```python
from build123d import *

# Parameters (mm, degrees)
SKETCH_1_W          = 24
SKETCH_1_H          = 40
SKETCH_1_R          = 2
EXTRUDE_1_DEPTH     = 5
EXTRUDE_5_DEPTH     = 67.34
SKETCH_10_W         = 10
SKETCH_10_H         = 28
EXTRUDE_6_DEPTH     = 18.5
SKETCH_12_R         = 2
CUT_EXTRUDE_4_DEPTH = 24.5
SKETCH_13_W         = 12
SKETCH_13_H         = 28
CUT_EXTRUDE_5_DEPTH = 2


with BuildPart() as part:
    # 草图1 → 凸台-拉伸1 (new body)
    with BuildSketch(Plane(origin=(0, 0, 0), x_dir=(1, 0, 0), z_dir=(0, 1, 0))):
        Rectangle(SKETCH_1_W, SKETCH_1_H)
        with Locations((7.5, -14.8)):
            Circle(SKETCH_1_R, mode=Mode.SUBTRACT)
        with Locations((-7.5, -14.8)):
            Circle(SKETCH_1_R, mode=Mode.SUBTRACT)
        with Locations((-7.5, 14.8)):
            Circle(SKETCH_1_R, mode=Mode.SUBTRACT)
        with Locations((7.5, 14.8)):
            Circle(SKETCH_1_R, mode=Mode.SUBTRACT)
    extrude(amount=EXTRUDE_1_DEPTH)

    # 草图8 → 凸台-拉伸5 (add)
    with BuildSketch(Plane(origin=(0, 5, 0), x_dir=(1, 0, 0), z_dir=(0, 1, 0))):
        Polygon((-5, 0), (-5, -20), (5, -20), (5, 20), (-5, 20), align=None)
    extrude(amount=EXTRUDE_5_DEPTH)

    # 草图10 → 凸台-拉伸6 (add)
    with BuildSketch(Plane(origin=(5, 0, 0), x_dir=(0, 0, -1), z_dir=(1, 0, 0))):
        with Locations((0, 58.34)):
            Rectangle(SKETCH_10_W, SKETCH_10_H)
    extrude(amount=EXTRUDE_6_DEPTH)

    # 草图12 → 切除-拉伸4 (cut)
    with BuildSketch(Plane(origin=(0, 0, -5), x_dir=(-1, 0, 0), z_dir=(0, 0, -1))):
        with Locations((-15.41, 68.31)):
            Circle(SKETCH_12_R)
        with Locations((-15.41, 58.49)):
            Circle(SKETCH_12_R)
        with Locations((-15.41, 48.67)):
            Circle(SKETCH_12_R)
    extrude(amount=-CUT_EXTRUDE_4_DEPTH, mode=Mode.SUBTRACT)

    # 草图13 → 切除-拉伸5 (cut, symmetric)
    with BuildSketch(Plane.XY):
        with Locations((17.5, 58.34)):
            Rectangle(SKETCH_13_W, SKETCH_13_H)
    extrude(amount=CUT_EXTRUDE_5_DEPTH, both=True, mode=Mode.SUBTRACT)


solid = part.part
```
Design review of the part built by this model. Coordinates are the model's own, in mm. A direction names the side the tool comes from. Coordinates: 2 decimals unless noted, no trailing zeros. Order: outer loops, then holes, each group sorted by start corner. A loop starts at its lowest first (then second) coordinate and runs counter-clockwise, first axis right, second up.
1) Wall thickness on line 1 along Z through (x, y) = (-7.5, 3.55); line 2 along Y through (x, z) = (15.41, 3.25); line 3 along Y through (x, z) = (9.5, 1): over which ranges is each line inside the solid? List them lowest first.
2) Take a section at B-B, the plane y = 68.31. Give the boundary of the cut face in (x, z), and give its area (3 significant figures).
3) Take a section at C-C, the plane z = 3.5. Give the boundary of the cut face in (x, y), and give its area (3 significant figures).
4) For faces 1 (the flat face through (12, 58, 5)), 2 (the flat face through (-9, 5, 0)), 3 (the flat face through (14.1, 44.34, -2.2)), 4 (the flat face through (12, 58, -5)), 5 (the flat face through (0, 28, -20)), list the 3-axis set-ups (+Z, -Z, +X, -X, +Y, -Y) from which the entire face can be reached by the end or side of a thin tool; tool diameter is ignored.
5) Clearance check with flat-ended pins moving along their axes: pin 1 (6.5 mm diameter, centred on x = 15.41, y = 68.31, fed in from +Z); pin 2 (5.5 mm diameter, centred on y = 2.5, z = -1.5, fed in from +X); pin 3 (5 mm diameter, centred on x = 15.41, y = 48.67, fed in from -Z); pin 4 (3.5 mm diameter, centred on x = 15.41, y = 58.49, fed in from -Z). State where each tip first meets the part, or that it passes through.
6) Mouldability with a two-part tool opening along Y and no side actions: class faces 6 (the flat face through (5, 38, 0)), 7 (the flat face through (23.5, 59, -3)), 8 (the flat face through (0, 0, 0)) as +Y half, -Y half, draft (parallel to the pull), parting line (faces both ways), or undercut.
7) Take a section at A-A, the plane x = 7.5. Give the boundary of the cut face in (y, z), and give its area (3 significant figures).
8) Take a section at D-D, the plane z = 14.8. Give the boundary of the cut face in (x, y).
Returned:
1. line 1: z = -20 to -16.8, -12.8 to 12.8, 16.8 to 20
1. line 2: y = 44.34 to 46.67, 50.67 to 56.49, 60.49 to 66.31, 70.31 to 72.34
1. line 3: y = 0 to 5, 44.34 to 72.34
2. outline: (-5, -20) - (5, -20) - (5, -5) - (13.41, -5) - (13.41, -2) - (11.5, -2) - (11.5, 2) - (13.41, 2) - (13.41, 5) - (5, 5) - (5, 20) - (-5, 20) - close; (17.41, -5) - (23.5, -5) - (23.5, -2) - (17.41, -2) - close; (17.41, 2) - (23.5, 2) - (23.5, 5) - (17.41, 5) - close
2. area: 513 mm2
3. outline: (-12, 0) - (12, 0) - (12, 5) - (5, 5) - (5, 44.34) - (23.5, 44.34) - (23.5, 72.34) - (-5, 72.34) - (-5, 5) - (-12, 5) - close; hole circle Ø4 at (15.41, 48.67); hole circle Ø4 at (15.41, 58.49); hole circle Ø4 at (15.41, 68.31)
3. area: 1,270 mm2
4. face 1: +Z, +X, +Y
4. face 2: +Z, -Z, -X, +Y
4. face 3: +Z, -Z, +X
4. face 4: -Z, +X, +Y
4. face 5: -Z, +X, -X, +Y, -Y
5. pin 1: stops at z = 5
5. pin 2: stops at x = 12
5. pin 3: stops at z = -5
5. pin 4: passes through
6. face 6: undercut
6. face 7: draft
6. face 8: -Y half
7. outline: (0, -20) - (5, -20) - (5, -16.8) - (0, -16.8) - close; (0, -12.8) - (5, -12.8) - (5, 12.8) - (0, 12.8) - close; (0, 16.8) - (5, 16.8) - (5, 20) - (0, 20) - close; (44.34, -5) - (72.34, -5) - (72.34, 5) - (44.34, 5) - close
7. area: 440 mm2
8. outline: (-12, 0) - (-9.5, 0) - (-9.5, 5) - (-12, 5) - close; (-5.5, 0) - (5.5, 0) - (5.5, 5) - (5, 5) - (5, 72.34) - (-5, 72.34) - (-5, 5) - (-5.5, 5) - close; (9.5, 0) - (12, 0) - (12, 5) - (9.5, 5) - close
